Verification items for the finished model (mm, model axes). A direction names the side the tool comes from. Give positions to 0.01 mm unless a question says otherwise; leave off trailing zeros. Order: outer loops, then holes, each group sorted by start corner. A loop starts at its lowest first (then second) coordinate and runs counter-clockwise, first axis right, second up.
(1) Sectioned sample at B-B on x = 9.25. Record the cut outline in (y, z), plus the area to 3 significant figures.
(2) Sectioned sample at C-C on y = 29. Record the cut outline in (x, z), plus the area to 3 significant figures.
(3) Sectioned sample at A-A on y = 53. Record the cut outline in (x, z), plus the area to 3 significant figures.
(4) Gauge pin test, flat ends, axial feed: pin 1 (3 mm diameter, centred on x = 8.5, z = -2, fed in from -Y); pin 2 (4 mm diameter, centred on x = 1, y = 51.5, fed in from +Z); pin 3 (3 mm diameter, centred on x = 8.5, z = -1.5, fed in from +Y); pin 4 (2 mm diameter, centred on x = 7, y = 27, fed in from -Z). Record the tip position at first contact, or that the pin passes through.
(5) Scan lines: L1, parallel to Y at x = -0.5, z = 6.75; L2, parallel to Y at x = 4.5, z = 2.75; L3, parallel to Y at x = 3.25, z = 2.25. Record each from-to range of solid material in increasing order.
(6) Mould release check, pull along Y, two halves, no side actions. Record for faces 1 (the face through (-5.2, 12.5, -0.1)), 2 (the face through (-2, 44, 2)), 3 (the face through (0, 0, 0)), 4 (the face through (-0.68, 68.68, -0.15)): pulls with the +Y half, pulls with the -Y half, needs draft (parallel to the pull), parting line crosses it, or undercut.
(7) Access from +Z, -Z, +X, -X, +Y, -Y to the whole of each face (thin tool, end or side, straight path). Record for faces 5 (the face through (10.885, 28.55, 2.417)), 6 (the face through (2, 64, 2)), 7 (the face through (-7.81, 2.46, -1.73)), 8 (the face through (-1.952, 43.493, -0.434)).
```python
from build123d import *

# Parameters (mm, degrees)
SKETCH1_R           = 8
BOSS_EXTRUDE1_DEPTH = 5
SKETCH2_R           = 6
BOSS_EXTRUDE2_DEPTH = 6
SKETCH3_R           = 8
BOSS_EXTRUDE3_DEPTH = 1.5
SKETCH4_R           = 5
BOSS_EXTRUDE4_DEPTH = 2
SKETCH5_R           = 11.15
BOSS_EXTRUDE5_DEPTH = 28.5
SKETCH6_R           = 2
BOSS_EXTRUDE6_DEPTH = 1
SKETCH7_R           = 8
BOSS_EXTRUDE7_DEPTH = 20
SKETCH8_R           = 2.5
BOSS_EXTRUDE8_DEPTH = 3
SKETCH9_R           = 2.5
BOSS_EXTRUDE9_DEPTH = 2
BOSS_EXTRUDE9_TAPER = 47


with BuildPart() as part:
    # Sketch1 → Boss-Extrude1 (new body)
    with BuildSketch(Plane(origin=(0, 0, 0), x_dir=(1, 0, 0), z_dir=(0, 1, 0))):
        with Locations(Location((0, 0, 0), (0, 0, 270))):
            Circle(SKETCH1_R)
    extrude(amount=BOSS_EXTRUDE1_DEPTH)

    # Sketch2 → Boss-Extrude2 (add)
    with BuildSketch(Plane(origin=(0, 5, 0), x_dir=(1, 0, 0), z_dir=(0, 1, 0))):
        with Locations(Location((0, 0, 0), (0, 0, 270))):
            Circle(SKETCH2_R)
    extrude(amount=BOSS_EXTRUDE2_DEPTH)

    # Sketch3 → Boss-Extrude3 (add)
    with BuildSketch(Plane(origin=(0, 11, 0), x_dir=(1, 0, 0), z_dir=(0, 1, 0))):
        with Locations(Location((0, 0, 0), (0, 0, 270))):
            Circle(SKETCH3_R)
    extrude(amount=BOSS_EXTRUDE3_DEPTH)

    # Sketch4 → Boss-Extrude4 (add)
    with BuildSketch(Plane(origin=(0, 12.5, 0), x_dir=(1, 0, 0), z_dir=(0, 1, 0))):
        with Locations(Location((0, 0, 0), (0, 0, 270))):
            Circle(SKETCH4_R)
    extrude(amount=BOSS_EXTRUDE4_DEPTH)

    # Sketch5 → Boss-Extrude5 (add)
    with BuildSketch(Plane(origin=(0, 14.5, 0), x_dir=(1, 0, 0), z_dir=(0, 1, 0))):
        with Locations(Location((0, 0, 0), (0, 0, 90))):
            Circle(SKETCH5_R)
    extrude(amount=BOSS_EXTRUDE5_DEPTH)

    # Sketch6 → Boss-Extrude6 (add)
    with BuildSketch(Plane(origin=(0, 43, 0), x_dir=(1, 0, 0), z_dir=(0, 1, 0))):
        with Locations(Location((0, 0, 0), (0, 0, 270))):
            Circle(SKETCH6_R)
    extrude(amount=BOSS_EXTRUDE6_DEPTH)

    # Sketch7 → Boss-Extrude7 (add)
    with BuildSketch(Plane(origin=(0, 44, 0), x_dir=(1, 0, 0), z_dir=(0, 1, 0))):
        with Locations(Location((0, 0, 0), (0, 0, 270))):
            Circle(SKETCH7_R)
    extrude(amount=BOSS_EXTRUDE7_DEPTH)

    # Sketch8 → Boss-Extrude8 (add)
    with BuildSketch(Plane(origin=(0, 64, 0), x_dir=(1, 0, 0), z_dir=(0, 1, 0))):
        with Locations(Location((0, 0, 0), (0, 0, 270))):
            Circle(SKETCH8_R)
    extrude(amount=BOSS_EXTRUDE8_DEPTH)

    # Sketch9 → Boss-Extrude9 (add)
    with BuildSketch(Plane(origin=(0, 67, 0), x_dir=(1, 0, 0), z_dir=(0, 1, 0))):
        with Locations(Location((0, 0, 0), (0, 0, 270))):
            Circle(SKETCH9_R)
    extrude(amount=BOSS_EXTRUDE9_DEPTH, taper=BOSS_EXTRUDE9_TAPER)


solid = part.part
```
Ans:
1. outline: (14.5, -6.23) - (43, -6.23) - (43, 6.23) - (14.5, 6.23) - close
1. area: 355 mm2
2. outline: circle Ø22.3 at (0, 0)
2. area: 391 mm2
3. outline: circle Ø16 at (0, 0)
3. area: 201 mm2
4. pin 1: stops at y = 0
4. pin 2: stops at z = 8
4. pin 3: stops at y = 64
4. pin 4: stops at z = -9.4
5. L1: y = 0 to 5, 11 to 12.5, 14.5 to 43, 44 to 64
5. L2: y = 0 to 12.5, 14.5 to 43, 44 to 64
5. L3: y = 0 to 43, 44 to 64
6. face 1: undercut
6. face 2: undercut
6. face 3: pulls with the -Y half
6. face 4: pulls with the +Y half
7. face 5: +Y, -Y
7. face 6: +Y
7. face 7: -Y
7. face 8: none
